from build123d import *

# Parameters (mm, degrees)
SKETCH1_W                     = 74
SKETCH1_H                     = 30
BOSS_EXTRUDE1_DEPTH           = 10
SKETCH2_R                     = 6.4
CUT_EXTRUDE1_DEPTH            = 15
BOSS_EXTRUDE2_DEPTH           = 30
M3_CLEARANCE_HOLE1_AT_2_COUNT = 2
M3_CLEARANCE_HOLE1_AT_2_PITCH = 20
CUT_EXTRUDE2_REACH            = 92.574
SKETCH10_W                    = 6.16
SKETCH10_H                    = 4
FILLET1_R                     = 1
CUT_EXTRUDE3_REACH            = 99.255


with BuildPart() as part:
    # Sketch1 → Boss-Extrude1 (new body)
    with BuildSketch(Plane(origin=(0, 0, 0), x_dir=(1, 0, 0), z_dir=(0, 1, 0))):
        with Locations((37, 15)):
            Rectangle(SKETCH1_W, SKETCH1_H)
    extrude(amount=BOSS_EXTRUDE1_DEPTH)

    # Sketch2 → Cut-Extrude1 (cut)
    with BuildSketch(Plane(origin=(0, 10, 0), x_dir=(1, 0, 0), z_dir=(0, 1, 0))):
        with Locations(Location((24.75, 15, 0), (0, 0, 270))):
            Circle(SKETCH2_R)
    extrude(amount=-CUT_EXTRUDE1_DEPTH, mode=Mode.SUBTRACT)

    # Sketch3 → Boss-Extrude2 (add)
    with BuildSketch(Plane.XY):
        Polygon((6, -40), (8, -40), (8, -42.75), (-2, -42.75), (-2, -40), (0, -40), (0, 0), (6, 0), align=None)
    boss_extrude2 = extrude(amount=-BOSS_EXTRUDE2_DEPTH)

    # Sketch9 → M3 Clearance Hole1 (revolve, cut)
    with BuildSketch(Plane(origin=(3, -42.75, -5), x_dir=(0, 0, -1), z_dir=(1, 0, 0))):
        Polygon((0, 0), (0, 11.081549114), (1.8, 10), (1.8, 0), align=None)
    m3_clearance_hole1 = revolve(axis=Axis((3, -49.1, -5), (0, 1, 0)), mode=Mode.SUBTRACT)

    # M3 Clearance Hole1 at 2: M3 Clearance Hole1 ×2
    with Locations(*[(0, 0, -i * M3_CLEARANCE_HOLE1_AT_2_PITCH) for i in range(1, M3_CLEARANCE_HOLE1_AT_2_COUNT)]):
        add(m3_clearance_hole1, mode=Mode.SUBTRACT)

    # Sketch10 → Cut-Extrude2 (cut, up to next)
    with BuildSketch(Plane.ZY, mode=Mode.PRIVATE) as cut_extrude2_sk1:
        with Locations((-25, -36.75)):
            Rectangle(SKETCH10_W, SKETCH10_H)
    cut_extrude2_tool1 = extrude(cut_extrude2_sk1.sketch, amount=-CUT_EXTRUDE2_REACH, mode=Mode.PRIVATE) & part.part
    # Sketch10 → Cut-Extrude2 (cut, up to next)
    with BuildSketch(Plane.ZY, mode=Mode.PRIVATE) as cut_extrude2_sk2:
        with Locations((-5, -36.75)):
            Rectangle(SKETCH10_W, SKETCH10_H)
    cut_extrude2_tool2 = extrude(cut_extrude2_sk2.sketch, amount=-CUT_EXTRUDE2_REACH, mode=Mode.PRIVATE) & part.part
    cut_extrude2_1 = cut_extrude2_tool1.solids().sort_by_distance((0, -36.75, -25))[0]
    add(cut_extrude2_1, mode=Mode.SUBTRACT)
    cut_extrude2_2 = cut_extrude2_tool2.solids().sort_by_distance((0, -36.75, -5))[0]
    add(cut_extrude2_2, mode=Mode.SUBTRACT)
    cut_extrude2 = cut_extrude2_1 + cut_extrude2_2  # Cut-Extrude2 as one shape, for the pattern or mirror that repeats it

    # Mirror1: Boss-Extrude2, M3 Clearance Hole1, Cut-Extrude2 across plane
    add(boss_extrude2.mirror(Plane.ZY.offset(-37)))
    add(m3_clearance_hole1.mirror(Plane.ZY.offset(-37)), mode=Mode.SUBTRACT)
    add(cut_extrude2.mirror(Plane.ZY.offset(-37)), mode=Mode.SUBTRACT)

    # Mirror1 copy 1 sketch → Mirror1 copy 1 (revolve, cut)
    with BuildSketch(Plane(origin=(71, -42.75, -25), x_dir=(0, 0, -1), z_dir=(-1, 0, 0))):
        Polygon((0, 0), (0, -11.081549114), (1.8, -10), (1.8, 0), align=None)
    revolve(axis=Axis((71, -49.1, -25), (0, -1, 0)), mode=Mode.SUBTRACT)

    # Fillet1
    fillet1_edges = [part.edges().sort_by_distance(p)[0] for p in [
        (74, -40, -15),
        (68, -40, -15),
        (6, -40, -15),
        (0, -40, -15),
    ]]
    fillet(fillet1_edges, radius=FILLET1_R)
    fillet1_2_edges = [part.edges().sort_by_distance(p)[0] for p in [
        (66, -41.375, 0),
        (66, -41.375, -30),
        (76, -41.375, 0),
        (76, -41.375, -30),
        (76, -40, -15),
        (66, -40, -15),
        (8, -41.375, 0),
        (8, -41.375, -30),
        (8, -40, -15),
        (-2, -41.375, -30),
        (-2, -41.375, 0),
        (-2, -40, -15),
        (74, -14.5, 0),
        (68, -19.5, 0),
        (68, -19.5, -30),
        (37, 0, 0),
        (6, -19.5, 0),
        (0, -14.5, 0),
        (74, 10, -15),
        (37, 10, 0),
        (0, 10, -15),
        (74, -14.5, -30),
        (0, -14.5, -30),
        (6, -19.5, -30),
        (37, 0, -30),
        (37, 10, -30),
        (6.292893219, -39.707106781, -30),
        (-0.292893219, -39.707106781, -30),
        (74.292893219, -39.707106781, -30),
        (-0.292893219, -39.707106781, 0),
        (6.292893219, -39.707106781, 0),
        (67.707106781, -39.707106781, -30),
        (67.707106781, -39.707106781, 0),
        (74.292893219, -39.707106781, 0),
    ]]
    fillet(fillet1_2_edges, radius=FILLET1_R - 0.0001)  # a hair under: the kernel refuses the full size

    # Sketch11 → Cut-Extrude3 (cut, up to next)
    with BuildSketch(Plane(origin=(0, 10, 0), x_dir=(1, 0, 0), z_dir=(0, 1, 0)), mode=Mode.PRIVATE) as cut_extrude3_sk1:
        with BuildLine():
            Line((44, 19.5), (56, 19.5))
            ThreePointArc((56, 19.5), (60.5, 15), (56, 10.5))
            Line((56, 10.5), (44, 10.5))
            ThreePointArc((44, 10.5), (39.5, 15), (44, 19.5))
        make_face()
    cut_extrude3_tool1 = extrude(cut_extrude3_sk1.sketch, amount=-CUT_EXTRUDE3_REACH, mode=Mode.PRIVATE) & part.part
    add(cut_extrude3_tool1.solids().sort_by_distance((50, 10, -15))[0], mode=Mode.SUBTRACT)


solid = part.part
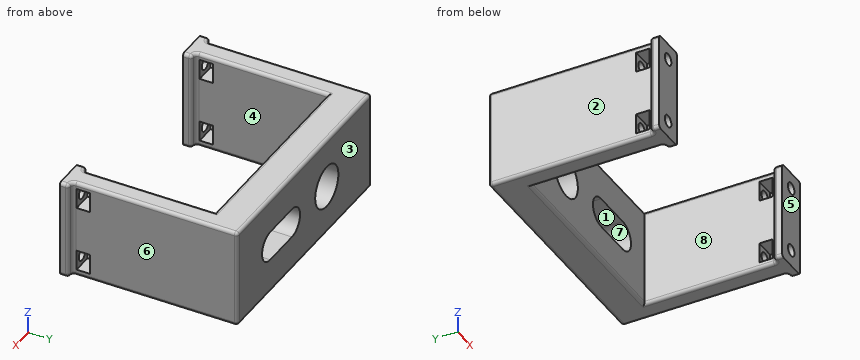
Model file for the job. Use its own axes, mm. Face numbers are marked on the shaded views. A direction names the side the tool comes from. Give positions to 0.01 mm unless a question says otherwise; leave off trailing zeros. Order: outer loops, then holes, each group sorted by start corner. A loop starts at its lowest first (then second) coordinate and runs counter-clockwise, first axis right, second up. Notation, with made-up numbers: (67.25, 88.25) - (90.25, 88.25) arc R22 ccw to (90.25, 116.25) - close; hole circle Ø11 at (8, 51). An arc over 180 degrees is marked (long way). Write item = value, one per line. Start each with the question number.
1. Probe line 1 along Z through (x, y) = (3, -34); line 2 along X through (y, z) = (-41.9, -25); line 3 along X through (y, z) = (7, -15). List the from-to ranges inside material, lowest first.
2. Cut at C-C, the plane z = -17.5. State how many separate pieces and enclosed holes the cut face has, and give its area (3 significant figures).
3. Cut at A-A, the plane y = -3. List the corners of the cut face in (x, z).
4. Drop flat-ended pins along their axis: P1, Ø10, axis at y = -3, z = -10, coming from the -X side; P2, Ø14, axis at y = -22, z = -20, coming from the +X side; P3, Ø4, axis at x = 41, y = -2.5, coming from the +Z side. Give the stop position or say it passes through.
5. Two-plate mould, pull along X, no slides. Class the marked faces 1, 2, 3 and 4: pulls with the +X half, pulls with the -X half, needs draft (parallel to the pull), parting line crosses it, or undercut.
6. Cut at D-D, the plane x = 38.5. List the corners of the cut face in (y, z).
7. Which spindle directions (+Z, -Z, +X, -X, +Y, -Y) get a long thin tool onto all of the face, cutting with end or side? Do the marked faces 5, 6, 7 and 8. Say none if no direction does.
8. Cut at B-B, the plane x = 24.75. List the corners of the cut face in (y, z), and give its area (3 significant figures).
Taken from the geometry:
q1.line_1 = -30 to -26.8, -23.2 to -6.8, -3.2 to 0
q1.line_2 = -2 to 1.2, 4.8 to 8, 66 to 69.2, 72.8 to 76
q1.line_3 = 0 to 18.35, 31.15 to 39.5, 60.5 to 74
q2.separate_pieces = 3
q2.enclosed_holes = 0
q2.area = 962 mm²
q3.outline = (0, -29) arc R1 ccw to (1, -30) - (5, -30) arc R1 ccw to (6, -29) - (6, -1) arc R1 ccw to (5, 0) - (1, 0) arc R1 ccw to (0, -1) - close; (68, -29) arc R1 ccw to (69, -30) - (73, -30) arc R1 ccw to (74, -29) - (74, -1) arc R1 ccw to (73, 0) - (69, 0) arc R1 ccw to (68, -1) - close
q4.P1 = 0
q4.P2 = 74
q4.P3 = through
q5.face_1 = undercut
q5.face_2 = pulls with the -X half
q5.face_3 = needs draft
q5.face_4 = undercut
q6.outline = (0, -29) arc R1 ccw to (1, -30) - (9, -30) arc R1 ccw to (10, -29) - (10, -1) arc R1 ccw to (9, 0) - (1, 0) arc R1 ccw to (0, -1) - close
q7.face_5 = +Z, -Z, +X, -X, -Y
q7.face_6 = +Z, -Z, +X, +Y
q7.face_7 = +Y, -Y
q7.face_8 = +Z, -Z
q8.outline = (0, -29) arc R1 ccw to (1, -30) - (9, -30) arc R1 ccw to (10, -29) - (10, -21.4) - (0, -21.4) - close; (0, -8.6) - (10, -8.6) - (10, -1) arc R1 ccw to (9, 0) - (1, 0) arc R1 ccw to (0, -1) - close
q8.area = 171 mm²
